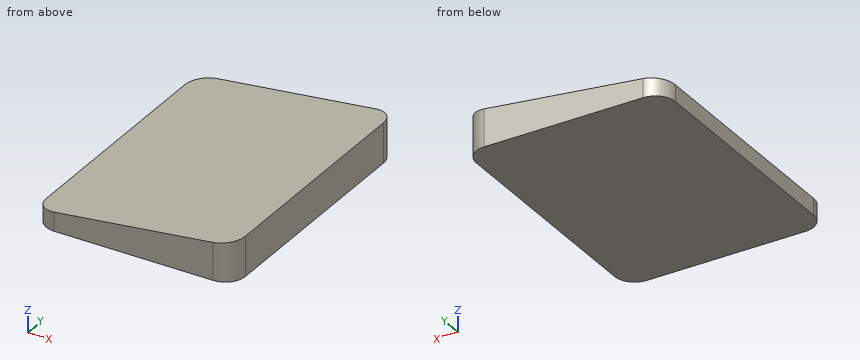
from build123d import *

# Parameters (mm, degrees)
F3_DEPTH = 15.24
F4_DEPTH = 304.801


with BuildPart() as f3:
    # F1 (on Top) → F3 (new body, through all)
    with BuildSketch(Plane.XY):
        with BuildLine():
            Line((30.48, 50.8), (-30.48, 50.8))
            ThreePointArc((-30.48, 50.8), (-35.868154, 48.568154), (-38.1, 43.18))
            Line((-38.1, 43.18), (-38.1, -43.18))
            ThreePointArc((-38.1, -43.18), (-35.868154, -48.568154), (-30.48, -50.8))
            Line((-30.48, -50.8), (30.48, -50.8))
            ThreePointArc((30.48, -50.8), (35.868154, -48.568154), (38.1, -43.18))
            Line((38.1, -43.18), (38.1, 43.18))
            ThreePointArc((38.1, 43.18), (35.868154, 48.568154), (30.48, 50.8))
        make_face()
    extrude(amount=F3_DEPTH)

    # F2 (on offset) → F4 (intersect, through all)
    with BuildSketch(Plane.XZ.offset(254)):
        Polygon((-38.1, 6.35), (-38.1, 0), (38.1, 0), (38.1, 15.24), align=None)
    extrude(amount=-F4_DEPTH, mode=Mode.INTERSECT)


solid = f3.part
Design review of the part built by this model. Coordinates are the model's own, in mm. Give positions to 0.01 mm unless a question says otherwise; leave off trailing zeros. Order: outer loops, then holes, each group sorted by start corner. A loop starts at its lowest first (then second) coordinate and runs counter-clockwise, first axis right, second up. Notation, with made-up numbers: (76, 84.25) - (132, 84.25) arc R15 ccw to (132, 110.25) - close; hole circle Ø10 at (47.25, 16.25). An arc over 180 degrees is marked (long way). Write item = value, one per line. Start each with the question number.
Q1. To check wall thickness, follow L1, parallel to Y at x = -31, z = 2.75; L2, parallel to Z at x = -21, y = 26 (3 decimals); L3, parallel to Z at x = -35, y = 12. State the ranges of each line that lie inside material, in increasing order. Write a range as from..to.
Q2. We need section C-C on x = -10.5. State the section outline as (y, z) points.
Q3. We need section A-A on z = 13. State the section outline as (x, y) points.
Q4. We need section B-B on y = 3.5. State the section outline as (x, z) points.
Q5. Clearance check with flat-ended pins moving along their axes: pin 1 Ø1.5 at (x, y) = (-4.5, 8) entering from -Z; pin 2 Ø2 at (x, y) = (-11, -20.5) entering from +Z; pin 3 Ø5 at (x, y) = (10.5, -1) entering from +Z; pin 4 Ø10 at (x, y) = (-18.5, -20) entering from +Z. State where each tip first meets the part, or that it passes through.
Working result:
q1.L1 = -50.78..50.78
q1.L2 = 0..8.345
q1.L3 = 0..6.71
q2.outline = (-50.8, 0) - (50.8, 0) - (50.8, 9.57) - (-50.8, 9.57) - close
q3.outline = (18.9, -50.8) - (30.48, -50.8) arc R7.62 ccw to (38.1, -43.18) - (38.1, 43.18) arc R7.62 ccw to (30.48, 50.8) - (18.9, 50.8) - close
q4.outline = (-38.1, 0) - (38.1, 0) - (38.1, 15.24) - (-38.1, 6.35) - close
q5.pin_1 = 0
q5.pin_2 = 9.63
q5.pin_3 = 12.31
q5.pin_4 = 9.22
